Geometry: final body of the model. Coordinates: model frame, mm. Face numbers are marked on the shaded views. A direction names the side the tool comes from. Give positions to 0.01 mm unless a question says otherwise; leave off trailing zeros. Order: outer loops, then holes, each group sorted by start corner. A loop starts at its lowest first (then second) coordinate and runs counter-clockwise, first axis right, second up. Notation, with made-up numbers: (10.25, 18) - (46.25, 18) arc R19 cw to (46.25, 35) - close; hole circle Ø6 at (80, 59.5). An arc over 180 degrees is marked (long way). Use one line per item in the form item = value.
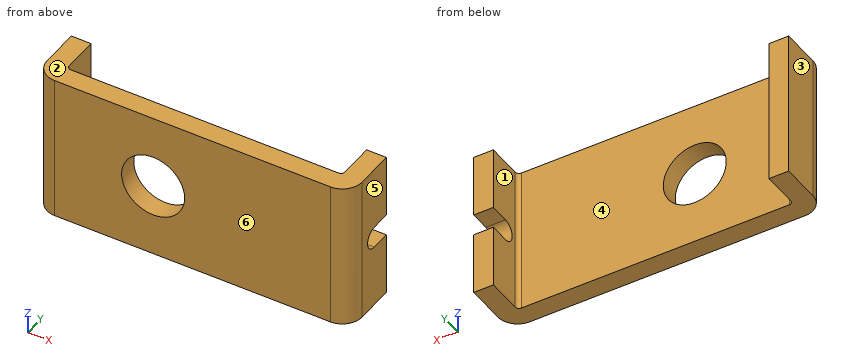
Autodesk Inventor part; units mm, degrees
ref_plane "YZ Plane" through (0, 0, 0) normal (1, 0, 0) x (0, 1, 0)
ref_plane "XZ Plane" through (0, 0, 0) normal (0, 1, 0) x (-1, 0, 0)
ref_plane "XY Plane" through (0, 0, 0) normal (0, 0, 1) x (1, 0, 0)
sketch "Sketch1" plane through (0, 0, 0) normal (0, 0, 1) x (1, 0, 0)
  line L0 (10, 0) -> (150, 0)
  line L1 (160, 0) -> (160, 30)
  line L2 (0, 10) -> (0, 30)
  line L3 (0, 30) -> (10, 30)
  line L4 (10, 30) -> (10, 10)
  line L5 (12, 10) -> (150, 10)
  line L6 (150, 12) -> (150, 30)
  line L7 (150, 30) -> (160, 30)
  arc A0 (0, 10) -> (10, 0) centre (10, 10) ccw
  arc A1 (150, 0) -> (160, 10) centre (150, 10) ccw
  arc A2 (10, 12) -> (12, 10) centre (12, 12) ccw
  arc A3 (148, 10) -> (150, 12) centre (148, 12) ccw
  point P0 (0, 0)
  dimension "d0" = 160
  dimension "d1" = 30
  dimension "d2" = 30
  dimension "d3" = 10
  dimension "d4" = 20
  dimension "d5" = 140
  dimension "d8" = 20
  dimension "d9" = 20
  dimension "d10" = 4
  dimension "d11" = 4
extrude "Extrusion1" add sketch "Sketch1" along normal mid plane 75
sketch "Sketch2" plane through (160, 10, 37.5) normal (1, 0, 0) x (0, 0, -1)
  line L0 (37.5, -10) -> (0, -10)
  line L1 (0, -10) -> (75, -10)
  line L2 (32, 20) -> (32, 10)
  line L3 (43, 20) -> (43, 10)
  arc A0 (32, 10) -> (43, 10) centre (37.5, 10) ccw
  line L4 (32, 20) -> (43, 20)
  line L5 (75, 20) -> (0, 20)
  dimension "d16" = 11
extrude "Extrusion2" cut sketch "Sketch2" against normal blind 75
sketch "Sketch3" plane through (12, 10, 37.5) normal (0, 1, 0) x (1, 0, 0)
  line L0 (0, 0) -> (0, 75)
  circle A0 centre (48, 37.5) radius 16
  line L1 (-12, 0) -> (-12, 75)
  line L2 (-12, 0) -> (-12, 37.5)
  line L3 (-12, 37.5) -> (48, 37.5)
  dimension "d20" = 32
  dimension "d22" = 60
extrude "Extrusion3" cut sketch "Sketch3" against normal through all
equation "\"BendRadius\" = Thickness"
equation "\"BendReliefWidth\" = Thickness"
equation "\"BendReliefDepth\" = 0.5 * Thickness"
equation "\"CornerReliefSize\" = 4 * Thickness"
equation "\"MinimumRemnant\" = 2 * Thickness"
equation "\"TransitionRadius\" = BendRadius"
equation "\"JacobiRadiusSize\" = BendRadius"
equation "\"GapSize\" = Thickness"
properties part number "Base-Plate"
(1) Reachability of the marked faces 1 and 2 from +Z, -Z, +X, -X, +Y, -Y: full face, straight path, thin tool, end or side. Return the list, or none.
Computed values:
face_1 = +Z, -Z, +Y
face_2 = +Z, +X, -X, +Y, -Y
(2) Pull-direction query (X, two-part tool) for the marked faces 3, 4, 5 and 6; classes: released by +X, released by -X, zero draft, split by the parting line, or undercut.
Computed values:
face_3 = released by -X
face_4 = undercut
face_5 = released by +X
face_6 = zero draft
(3) Cut plane C-C on z = 0. Output: boundary loops of the cut face in (x, y).
Computed values:
outline = (0, 10) arc R10 ccw to (10, 0) - (44, 0) - (44, 10) - (12, 10) arc R2 cw to (10, 12) - (10, 30) - (0, 30) - close; (76, 0) - (150, 0) arc R10 ccw to (160, 10) - (160, 14.5) - (150, 14.5) - (150, 12) arc R2 cw to (148, 10) - (76, 10) - close
(4) Cut plane A-A on x = 60. Output: boundary loops of the cut face in (y, z).
Computed values:
outline = (0, -37.5) - (10, -37.5) - (10, -16) - (0, -16) - close; (0, 16) - (10, 16) - (10, 37.5) - (0, 37.5) - close
(5) Ray query, line 1 along Z through (x, y) = (60, 6); line 2 along X through (y, z) = (28.5, 33); line 3 along Y through (x, z) = (70.5, 18.5). Return the intervals inside material, ascending.
Computed values:
line_1 = -37.5 to -16, 16 to 37.5
line_2 = 0 to 10, 150 to 160
line_3 = 0 to 10
(6) Contact query for flat-ended pins moving along their axis: pin 1 Ø10 at (x, z) = (116.5, -9.5) entering from +Y; pin 2 Ø2 at (y, z) = (3, 10) entering from -X. Output: stop coordinate, or through.
Computed values:
pin_1 = 10
pin_2 = 2
(7) Cut plane B-B on y = 26. Output: boundary loops of the cut face in (x, z), plus the area to 3 significant figures.
Computed values:
outline = (0, -37.5) - (10, -37.5) - (10, 37.5) - (0, 37.5) - close; (150, -37.5) - (160, -37.5) - (160, -5.5) - (150, -5.5) - close; (150, 5.5) - (160, 5.5) - (160, 37.5) - (150, 37.5) - close
area = 1,390 mm²
(8) Cut plane D-D on z = 19.5. Output: boundary loops of the cut face in (x, y).
Computed values:
outline = (0, 10) arc R10 ccw to (10, 0) - (150, 0) arc R10 ccw to (160, 10) - (160, 30) - (150, 30) - (150, 12) arc R2 cw to (148, 10) - (12, 10) arc R2 cw to (10, 12) - (10, 30) - (0, 30) - close
